```python
from build123d import *

# Parameters (mm, degrees)
BOSS_EXTRUDE2_DEPTH = 40
SKETCH3_W           = 3
SKETCH3_H           = 3
CUT_EXTRUDE2_DEPTH  = 45.805132264


with BuildPart() as part:
    # Sketch1 → Boss-Extrude2 (new, symmetric)
    with BuildSketch(Plane.XY):
        with BuildLine():
            ThreePointArc((0, 2.5), (-2.392060476, -0.726668205), (1.390587434, -2.077562656))
            ThreePointArc((1.390587434, -2.077562656), (1.797326731, -1.834582069), (2.226834249, -1.634582786))
            ThreePointArc((2.226834249, -1.634582786), (10.992934155, 0.492745515), (20, 0))
            ThreePointArc((20, 0), (10.143001238, 2.394009907), (0, 2.5))
        make_face()
    extrude(amount=BOSS_EXTRUDE2_DEPTH, both=True)

    # Sketch3 → Cut-Extrude2 (cut, through all)
    with BuildSketch(Plane(origin=(0, 0, 0), x_dir=(1, 0, 0), z_dir=(0, 1, 0))):
        with Locations((4.5, -13.5)):
            Rectangle(SKETCH3_W, SKETCH3_H)
        with Locations((4.5, 13.5)):
            Rectangle(SKETCH3_W, SKETCH3_H)
    extrude(amount=CUT_EXTRUDE2_DEPTH, mode=Mode.SUBTRACT)


solid = part.part
```
Here's how the part is built. I have some questions about the finished solid (model axes, mm). A direction names the side the tool comes from. Give positions to 0.01 mm unless a question says otherwise; leave off trailing zeros. Write each loop counter-clockwise with the first axis right and the second up, starting at its lowest first coordinate (ties: lowest second). Pieces come first, ordered by that corner, then holes. Notation, with made-up numbers: M 30.25,-11 L 55.25,-11 A26 ccw 55.25,7 Z; hole C -39,17.5 d5. An arc over 180 degrees is marked long. Put each result on its own line as item: value. Start each with the question number.
Item 1: Will these pins go through, and if not, where does the flat tip stop? pin 1 (1.4 mm diameter, centred on y = 1.5, z = 14, fed in from -X); pin 2 (1 mm diameter, centred on x = 0, z = -10.5, fed in from +Y); pin 3 (1.4 mm diameter, centred on y = 1, z = -14, fed in from -X).
Item 2: If we section it at C-C, the plane x = 17.25: Write out the boundary of the cut face in (y, z).
Item 3: If we section it at A-A, the plane y = 1.55: Write out the boundary of the cut face in (x, z), then the cut area to 3 significant figures.
Item 4: I need wall thicknesses on L1, parallel to Z at x = 4.75, y = 1.5; L2, parallel to X at y = -1.95, z = 3; L3, parallel to Y at x = -1.5, z = 31. Which ranges of each line are inside material? Lowest first, please. Write a range as from..to.
Item 5: If we section it at B-B, the plane z = -27: Write out the boundary of the cut face in (x, y) (1 decimal), then the cut area to 3 significant figures.
Item 6: On a 3-axis mill with a long thin cutter (end or side, diameter ignored), from which of +Z, -Z, +X, -X, +Y, -Y can I reach the whole of each face in a straight line? I mean faces 4 (the flat face through (3, 1, 14)), 5 (the cylindrical face through (10.284, 2.376, 0.56)). Say none if no direction works.
Item 7: Thinking about a two-plate mould opening in Z: for faces 1 (the flat face through (4, 1, 40)), 2 (the cylindrical face through (10.87, 0.48, 0.56)), 3 (the flat face through (4, 1, 12)), which applies, +Z half, -Z half, draft (parallel to the pull), parting line (faces both ways), or undercut?
Values:
1. pin 1: x = -2.37
1. pin 2: y = 2.55
1. pin 3: x = -2.48
2. outline: M 0.43,-40 L 0.91,-40 L 0.91,40 L 0.43,40 Z
3. outline: M -1.96,-40 L 14.84,-40 L 14.84,40 L -1.96,40 Z; hole M 3,-15 L 6,-15 L 6,-12 L 3,-12 Z; hole M 3,12 L 6,12 L 6,15 L 3,15 Z
3. area: 1,330 mm²
4. L1: -40..-15, -12..12, 15..40
4. L2: -1.56..1.59
4. L3: -2..2
5. outline: M 0,2.5 A2.5 ccw long 1.4,-2.1 A4.6 cw 2.2,-1.6 A30.9 cw 20,0 A44.6 ccw Z
5. area: 54.0 mm²
6. face 4: +Y
6. face 5: +Z, -Z, +Y
7. face 1: +Z half
7. face 2: draft
7. face 3: undercut
